Build history of the part. All positions in model axes, mm. Give positions to 0.01 mm unless a question says otherwise; leave off trailing zeros. Order: outer loops, then holes, each group sorted by start corner. A loop starts at its lowest first (then second) coordinate and runs counter-clockwise, first axis right, second up. Notation, with made-up numbers: (77, 10) -> (111, 10) arc R18 cw to (111, 23) -> close; hole circle Ø11 at (-9.75, 84). An arc over 180 degrees is marked (long way). One line per question, with ' | ' between items. Start each with the question number.
(1) Cut at B-B (y = 139.7). Give the cut face in (x, z), then the cut area to 3 significant figures.
(2) Cut at A-A (x = 254). Give the cut face in (y, z), then the cut area to 3 significant figures.
(3) Drill centre lines: L1, parallel to X at y = 254, z = 2.75; L2, parallel to Y at x = 12.7, z = 2; L3, parallel to Y at x = 431.8, z = 1.75. Where is each one in solid material? Low to high. Write a range as from..to.
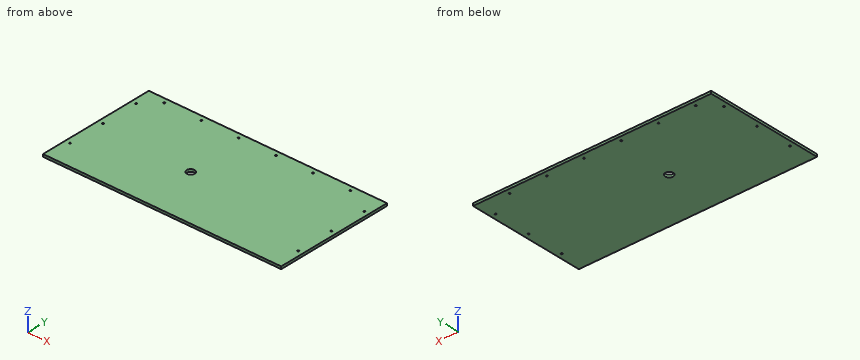
from build123d import *

# Parameters (mm, degrees)
SKETCH1_W           = 609.6
SKETCH1_H           = 304.8
BOSS_EXTRUDE1_DEPTH = 6.35
SKETCH2_R           = 2.032
CUT_EXTRUDE4_DEPTH  = 7.35
SKETCH4_R           = 2.032
CUT_EXTRUDE7_DEPTH  = 7.35
SKETCH5_R           = 10.16
CUT_EXTRUDE8_DEPTH  = 7.35


with BuildPart() as part:
    # Sketch1 → Boss-Extrude1 (new body)
    with BuildSketch(Plane.XY):
        with Locations((304.8, 152.4)):
            Rectangle(SKETCH1_W, SKETCH1_H)
    extrude(amount=BOSS_EXTRUDE1_DEPTH)

    # Sketch2 → Cut-Extrude4 (cut, through all)
    with BuildSketch(Plane.XY.offset(6.35)):
        with Locations((12.7, 254)):
            Circle(SKETCH2_R)
        with Locations((12.7, 158.75)):
            Circle(SKETCH2_R)
        with Locations((12.7, 63.5)):
            Circle(SKETCH2_R)
        with Locations((596.9, 63.5)):
            Circle(SKETCH2_R)
        with Locations((596.9, 158.75)):
            Circle(SKETCH2_R)
        with Locations((596.9, 254)):
            Circle(SKETCH2_R)
    extrude(amount=-CUT_EXTRUDE4_DEPTH, mode=Mode.SUBTRACT)

    # Sketch4 → Cut-Extrude7 (cut, through all)
    with BuildSketch(Plane.XY.offset(6.35)):
        with Locations((50.8, 292.1)):
            Circle(SKETCH4_R)
        with Locations((146.05, 292.1)):
            Circle(SKETCH4_R)
        with Locations((241.3, 292.1)):
            Circle(SKETCH4_R)
        with Locations((336.55, 292.1)):
            Circle(SKETCH4_R)
        with Locations((431.8, 292.1)):
            Circle(SKETCH4_R)
        with Locations((527.05, 292.1)):
            Circle(SKETCH4_R)
    extrude(amount=-CUT_EXTRUDE7_DEPTH, mode=Mode.SUBTRACT)

    # Sketch5 → Cut-Extrude8 (cut, through all)
    with BuildSketch(Plane(origin=(0, 0, 0), x_dir=(-1, 0, 0), z_dir=(0, 0, -1))):
        with Locations((-254, 139.7)):
            Circle(SKETCH5_R)
    extrude(amount=-CUT_EXTRUDE8_DEPTH, mode=Mode.SUBTRACT)


solid = part.part
Result set:
1) outline: (0, 0) -> (243.84, 0) -> (243.84, 6.35) -> (0, 6.35) -> close; (264.16, 0) -> (609.6, 0) -> (609.6, 6.35) -> (264.16, 6.35) -> close | area: 3,740 mm2
2) outline: (0, 0) -> (129.54, 0) -> (129.54, 6.35) -> (0, 6.35) -> close; (149.86, 0) -> (304.8, 0) -> (304.8, 6.35) -> (149.86, 6.35) -> close | area: 1,810 mm2
3) L1: x = 0..10.67, 14.73..594.87, 598.93..609.6 | L2: y = 0..61.47, 65.53..156.72, 160.78..251.97, 256.03..304.8 | L3: y = 0..290.07, 294.13..304.8
